Geometry: final body of the model. Coordinates: model frame, mm. Round coordinates to 2 decimals unless told otherwise and drop trailing zeros. Loops run counter-clockwise (first coordinate to the right, second up) from the corner with the lowest first, then second, coordinate; pieces in that order, holes last. Notation, with made-up numbers: (67, 32.25) - (97, 32.25) arc R30 cw to (97, 70.25) - close; hole circle Ø3 at (15.5, 73.25). An arc over 180 degrees is marked (long way). Use CSV: the item, a comma, the result in double quotes.
from build123d import *

# Parameters (mm, degrees)
SKETCH1_W               = 992
SKETCH1_H               = 746
BASE_FLANGE1_DEPTH      = 2
EDGE_FLANGE1_DEPTH      = 746
EDGE_FLANGE1_BEND_DEPTH = 746


# Sheet-metal steps are written as plain solids
with BuildPart() as part:
    # Sketch1 → Base-Flange1 (new body)
    with BuildSketch(Plane.YZ):
        Rectangle(SKETCH1_W, SKETCH1_H)
    extrude(amount=-BASE_FLANGE1_DEPTH)

    # Edge-Flange1 section (across the edge) → Edge-Flange1 (add)
    with BuildSketch(Plane(origin=(0, 498, -373), x_dir=(0, -1, 0), z_dir=(0, 0, 1))):
        with BuildLine():
            Line((-2, 2), (-2, 247))
            Line((-2, 247), (0, 247))
            Line((0, 247), (0, 2))
            ThreePointArc((0, 2), (0.585786438, 0.585786438), (2, 0))
            Line((2, 0), (2, -2))
            ThreePointArc((2, -2), (-0.828427125, -0.828427125), (-2, 2))
        make_face()
    extrude(amount=EDGE_FLANGE1_DEPTH)

    # Edge-Flange1 section 2 (across the edge) → Edge-Flange1 bend (add)
    with BuildSketch(Plane(origin=(0, -498, 373), x_dir=(0, 1, 0), z_dir=(0, 0, -1))):
        with BuildLine():
            Line((-2, 2), (-2, 247))
            Line((-2, 247), (0, 247))
            Line((0, 247), (0, 2))
            ThreePointArc((0, 2), (0.585786438, 0.585786438), (2, 0))
            Line((2, 0), (2, -2))
            ThreePointArc((2, -2), (-0.828427125, -0.828427125), (-2, 2))
        make_face()
    extrude(amount=EDGE_FLANGE1_BEND_DEPTH)


solid = part.part
Item 1: Section B-B on z = -99. Return the cut outline in (x, y), plus the area to 3 significant figures.
Final values:
outline,"(-2, -496) arc R4 ccw to (2, -500) - (247, -500) - (247, -498) - (2, -498) arc R2 cw to (0, -496) - (0, 496) arc R2 cw to (2, 498) - (247, 498) - (247, 500) - (2, 500) arc R4 ccw to (-2, 496) - close"
area,"2,980 mm²"
Item 2: Section A-A on x = 229. Return the cut outline in (y, z).
Final values:
outline,"(-500, -373) - (-498, -373) - (-498, 373) - (-500, 373) - close; (498, -373) - (500, -373) - (500, 373) - (498, 373) - close"
Item 3: Section C-C on y = -112. Return the cut outline in (x, z).
Final values:
outline,"(-2, -373) - (0, -373) - (0, 373) - (-2, 373) - close"
Item 4: Mould query, pull axis Y, two halves, no side actions, for faces 1 (the flat face through (123, -500, 5)), 2 (the flat face through (123, 500, -5)), 3 (the flat face through (126, -498, 5)), 4 (the flat face through (-2, -7, 5)). Classes: released by +Y, released by -Y, zero draft, split by the parting line, or undercut.
Final values:
face 1,"released by -Y"
face 2,"released by +Y"
face 3,"undercut"
face 4,"zero draft"
Item 5: Material intervals for line 1 (Y direction, x = 158.5, z = 25); line 2 (X direction, y = -142, z = 245), sorted ascending.
Final values:
line 1,"y = -500 to -498, 498 to 500"
line 2,"x = -2 to 0"
Item 6: Pin query (flat end, axial travel): P1, Ø8, axis at y = -274.5, z = 96, coming from the +X side. Return the tip coordinate at first contact, or that it passes through.
Final values:
P1,"stops at x = 0"
